```python
from build123d import *

# Parameters (mm, degrees)
F1_DEPTH = 50.8
F3_D     = 6.7564
F4_R     = 38.1
F5_DEPTH = 13.462
F6_R     = 12.7
F7_R     = 12.7
F8_SIZE  = 0.762
F10_D    = 6.5278


with BuildPart() as f1:
    # F0 (on Top) → F1 (new body, symmetric)
    with BuildSketch(Plane.XY):
        Polygon((0, -42.8148043404), (0, 58.7851956596), (-12.7, 58.7851956596), (-12.7, -46.8190989592), (19.8412804977, -93.2928638389), (30.2445114602, -86.0084430972), (29.1376829666, -84.4277281903), align=None)
    extrude(amount=F1_DEPTH, both=True)

    # F3 (through all)
    with Locations(Plane.YZ):
        with Locations((38.9459957701, 33.3375), (38.9459957701, -33.3375), (-21.1250042299, -33.3375), (-21.1250042299, 33.3375)):
            Hole(F3_D / 2)

    # F4 (on face) → F5 (cut)
    with BuildSketch(Plane.YZ):
        with Locations((8.7980022654, 0)):
            Circle(F4_R)
    extrude(amount=-F5_DEPTH, mode=Mode.SUBTRACT)

    # F6
    f6_edges = [f1.edges().sort_by_distance(p)[0] for p in [
        (-6.35, 58.785196, -50.8),
        (-6.35, 58.785196, 50.8),
        (25.042896, -89.650653, 50.8),
        (25.042896, -89.650653, -50.8),
    ]]
    fillet(f6_edges, radius=F6_R)

    # F7
    f7_edges = [f1.edges().sort_by_distance(p)[0] for p in [
        (0, -42.814804, 0),
        (-12.7, -46.819099, 0),
    ]]
    fillet(f7_edges, radius=F7_R)

    # F8
    f8_edges = [f1.edges().sort_by_distance(p)[0] for p in [
        (0, -29.301998, 0),
        (-12.7, -29.301998, 0),
        (0, 58.785196, 0),
        (0, 55.065452, -47.080256),
        (0, 3.637343, -50.8),
        (0.587795, -42.629473, -50.8),
        (28.110954, -82.961407, -47.080256),
        (12.62843, -60.850071, -50.8),
        (30.244511, -86.008443, 0),
        (28.110954, -82.961407, 47.080256),
        (12.62843, -60.850071, 50.8),
        (-12.7, 55.065452, 47.080256),
        (-12.7, 1.635196, 50.8),
        (-12.7, 58.785196, 0),
    ]]
    chamfer(f8_edges, length=F8_SIZE)

    # F10 (through all)
    with Locations(Plane(origin=(-20.1163778496, -14.0856394117, 0), x_dir=(-0.5735764364, 0.8191520443, 0), z_dir=(0.8191520443, 0.5735764364, 0))):
        with Locations((-57.15, -26.19375), (-57.15, 26.19375)):
            Hole(F10_D / 2)


solid = f1.part
```
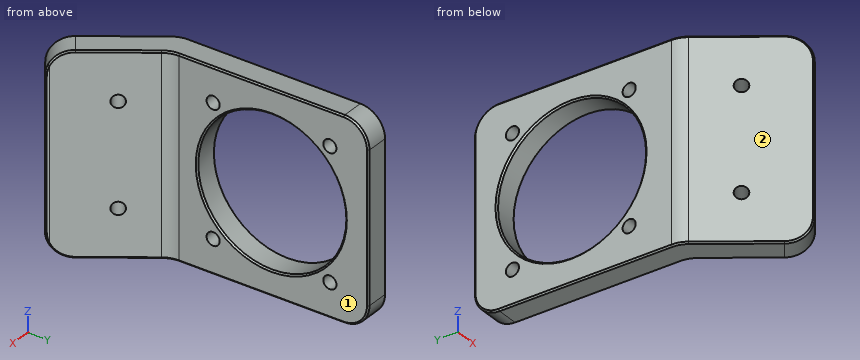
Check sheet for the modelled part. Datum: model origin and axes. Units: mm. Face numbers are marked on the shaded views. A direction names the side the tool comes from. Round coordinates to 2 decimals unless told otherwise and drop trailing zeros. Write each loop counter-clockwise with the first axis right and the second up, starting at its lowest first coordinate (ties: lowest second). Pieces come first, ordered by that corner, then holes. Notation, with made-up numbers: M 35,5 L 90,5 A16 ccw 90,27 Z; hole C -2.5,-32 d6. An arc over 180 degrees is marked long. Write item = value, one per line. Start each with the question number.
1. Section check C-C, the plane y = -32.5. Record the cut outline in (x, z), then the cut area to 3 significant figures.
2. Scan lines: line 1 (Z direction, x = -0.5, y = 10.5); line 2 (X direction, y = -30.5, z = -26); line 3 (Y direction, x = -4, z = 11). Record each from-to range of solid material in increasing order. Write a range as [from, to].
3. Gauge pin test, flat ends, axial feed: pin 1 (6 mm diameter, centred on x = 11.5, z = -20, fed in from -Y); pin 2 (1.5 mm diameter, centred on x = 12, z = -35, fed in from -Y); pin 3 (8 mm diameter, centred on x = 11.5, z = 10, fed in from +Y); pin 4 (6 mm diameter, centred on y = -21.13, z = -33.34, fed in from +X). Record the tip position at first contact, or that the pin passes through.
4. Section check B-B, the plane x = -4.5. Record the cut outline in (y, z) (1 decimal), then the cut area to 3 significant figures.
5. Section check A-A, the plane z = 0. Record the cut outline in (x, y), then the cut area to 3 significant figures.
6. Tool access check on the marked faces 1 and 2. Record the directions out of +Z, -Z, +X, -X, +Y, -Y that give a thin tool (end or side, any length) a straight path to the whole face; none if there is none.
7. Section check D-D, the plane y = -52.5. Record the cut outline in (x, z), then the cut area to 3 significant figures.
Results found:
q1.outline = M -12.7,-50.04 L -11.94,-50.8 L -0.76,-50.8 L 0,-50.04 L 0,50.04 L -0.76,50.8 L -11.94,50.8 L -12.7,50.04 Z
q1.area = 1,290 mm^2
q2.line_1 = [-50.54, -38.32], [38.32, 50.54]
q2.line_2 = [-12.7, 0]
q2.line_3 = [-59.24, -27.68], [45.28, 58.79]
q3.pin_1 = -85.66
q3.pin_2 = -83.17
q3.pin_3 = -53.53
q3.pin_4 = through
q4.outline = M -58.5,-50 L -57.2,-50.8 L 46.1,-50.8 A12.7 ccw 58.8,-38.1 L 58.8,38.1 A12.7 ccw 46.1,50.8 L -57.2,50.8 L -58.5,50 Z; hole C 8.8,0 d76.2; hole C -21.1,-33.3 d6.8; hole C -21.1,33.3 d6.8; hole C 38.9,-33.3 d6.8; hole C 38.9,33.3 d6.8
q4.area = 7,150 mm^2
q5.outline = M -12.7,-42.81 A12.7 ccw -10.4,-50.1 L 19.4,-92.67 L 20.47,-92.86 L 29.62,-86.45 L 29.81,-85.38 L 2.3,-46.09 A12.7 cw 0,-38.81 L 0,-30.06 L -0.76,-29.3 L -11.94,-29.3 L -12.7,-30.06 Z; M -12.7,47.66 L -11.94,46.9 L -0.76,46.9 L 0,47.66 L 0,58.02 L -0.76,58.79 L -11.94,58.79 L -12.7,58.02 Z
q5.area = 1,040 mm^2
q6.face_1 = +Z, -Z, +X, +Y
q6.face_2 = +Z, -Z, -X, -Y
q7.outline = M -8.72,-50.04 L -7.79,-50.8 L 5.85,-50.8 L 6.78,-50.04 L 6.78,50.04 L 5.85,50.8 L -7.79,50.8 L -8.72,50.04 Z
q7.area = 1,570 mm^2
